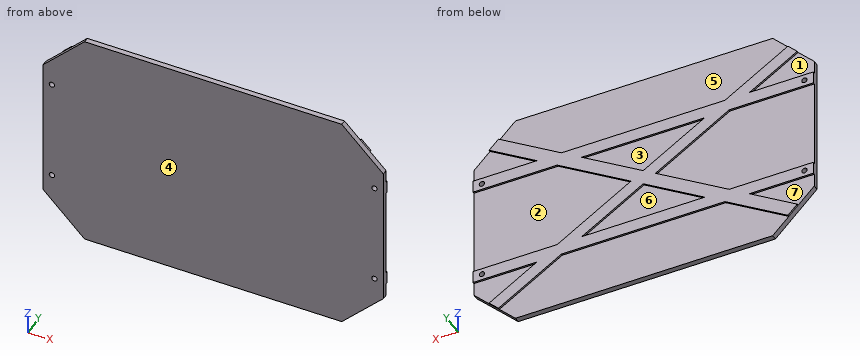
from build123d import *

# Parameters (mm, degrees)
SALIENTE_EXTRUIR1_DEPTH = 3
SALIENTE_EXTRUIR2_DEPTH = 1
CROQUIS3_R              = 1.5
CORTAR_EXTRUIR1_DEPTH   = 115.662203643
CROQUIS5_R              = 1.5
CORTAR_EXTRUIR2_DEPTH   = 115.662203643


with BuildPart() as part:
    # Croquis1 → Saliente-Extruir1 (new body)
    with BuildSketch(Plane(origin=(0, 0, 0), x_dir=(1, 0, 0), z_dir=(0, 1, 0))):
        Polygon((-72.165, -63.334523779), (72.165, -63.334523779), (95.499523779, -40), (95.499523779, 40), (72.165, 63.334523779), (-72.165, 63.334523779), (-95.499523779, 40), (-95.499523779, -40), align=None)
    extrude(amount=SALIENTE_EXTRUIR1_DEPTH)

    # Croquis2 → Saliente-Extruir2 (add)
    with BuildSketch(Plane(origin=(0, 3, 0), x_dir=(1, 0, 0), z_dir=(0, 1, 0))):
        Polygon((-95.499523779, -25.5), (-95.499523779, -32.5), (-59.599057268, -32.5), (-86.448609178, -49.046390822), (-81.218176491, -54.281347289), (-45.874561104, -32.5), (45.875356635, -32.5), (81.215914601, -54.279085399), (86.450579917, -49.048363047), (59.59824255, -32.5), (95.499523779, -32.5), (95.499523779, -25.5), (48.239634992, -25.5), (6.861850317, 0), (48.239634992, 25.5), (95.499523779, 25.5), (95.499523779, 32.5), (59.59824255, 32.5), (86.450579917, 49.048363047), (81.215914601, 54.279085399), (45.875356635, 32.5), (-45.874561104, 32.5), (-81.218176491, 54.281347289), (-86.448609178, 49.046390822), (-59.599057268, 32.5), (-95.499523779, 32.5), (-95.499523779, 25.5), (-48.240274232, 25.5), (-6.861850317, 0), (-48.240274232, -25.5), align=None)
        Polygon((34.516573599, -25.5), (-34.515975042, -25.5), (0, -4.228705845), align=None, mode=Mode.SUBTRACT)
        Polygon((0, 4.228705845), (-34.515975042, 25.5), (34.516573599, 25.5), align=None, mode=Mode.SUBTRACT)
    extrude(amount=SALIENTE_EXTRUIR2_DEPTH)

    # Croquis3 → Cortar-Extruir1 (cut, through all)
    with BuildSketch(Plane(origin=(0, 4, 0), x_dir=(1, 0, 0), z_dir=(0, 1, 0))):
        with Locations(Location((-90.499523779, -29, 0), (0, 0, 270))):
            Circle(CROQUIS3_R)
    extrude(amount=-CORTAR_EXTRUIR1_DEPTH, mode=Mode.SUBTRACT)

    # Croquis5 → Cortar-Extruir2 (cut, through all)
    with BuildSketch(Plane(origin=(0, 4, 0), x_dir=(1, 0, 0), z_dir=(0, 1, 0))):
        with Locations(Location((-90.499523779, 29, 0), (0, 0, 270))):
            Circle(CROQUIS5_R)
        with Locations(Location((90.499523779, 29, 0), (0, 0, 270))):
            Circle(CROQUIS5_R)
        with Locations(Location((90.499523779, -29, 0), (0, 0, 270))):
            Circle(CROQUIS5_R)
    extrude(amount=-CORTAR_EXTRUIR2_DEPTH, mode=Mode.SUBTRACT)


solid = part.part
Source: CAD feature listing. Evaluate the final solid. Frame: model axes, mm. Face numbers are marked on the shaded views. A direction names the side the tool comes from. Round coordinates to 2 decimals unless told otherwise and drop trailing zeros. Order: outer loops, then holes, each group sorted by start corner. A loop starts at its lowest first (then second) coordinate and runs counter-clockwise, first axis right, second up. Notation, with made-up numbers: (-37.75, 5) -> (16.25, 5) arc R23 ccw to (16.25, 31) -> close; hole circle Ø11 at (-35.75, 82). An arc over 180 degrees is marked (long way). Answer as CSV lines item,"result".
Item 1: Reachability of the marked faces 1, 2, 3 and 4 from +Z, -Z, +X, -X, +Y, -Y: full face, straight path, thin tool, end or side. Return the list, or none.
A:
face 1,"-X, +Y"
face 2,"+X, +Y"
face 3,"+Y"
face 4,"+Z, -Z, +X, -X, -Y"
Item 2: Line query: L1, parallel to X at y = 0.8, z = -29; L2, parallel to Z at x = 13.5, y = 3.7; L3, parallel to X at y = 2.7, z = 30. Output: solid intervals per line, ascending.
A:
L1,"-95.5 to -92, -89 to 89, 92 to 95.5"
L2,"-32.5 to -25.5, -12.55 to -4.09, 4.09 to 12.55, 25.5 to 32.5"
L3,"-95.5 to -91.62, -89.38 to 89.38, 91.62 to 95.5"
Item 3: Section A-A, the plane x = -69. Return loops of the section in (y, z).
A:
outline,"(0, -63.33) -> (3, -63.33) -> (3, -46.75) -> (4, -46.75) -> (4, -38.29) -> (3, -38.29) -> (3, -32.5) -> (4, -32.5) -> (4, -25.5) -> (3, -25.5) -> (3, 25.5) -> (4, 25.5) -> (4, 32.5) -> (3, 32.5) -> (3, 38.29) -> (4, 38.29) -> (4, 46.75) -> (3, 46.75) -> (3, 63.33) -> (0, 63.33) -> close"
Item 4: Pull-direction query (X, two-part tool) for the marked faces 5, 6 and 7; classes: pulls with the +X half, pulls with the -X half, needs draft (parallel to the pull), parting line crosses it, or undercut.
A:
face 5,"undercut"
face 6,"undercut"
face 7,"needs draft"
Item 5: Section B-B, the plane y = 1.55. Return loops of the section in (x, z) (3 decimals).
A:
outline,"(-95.5, -40) -> (-72.165, -63.335) -> (72.165, -63.335) -> (95.5, -40) -> (95.5, 40) -> (72.165, 63.335) -> (-72.165, 63.335) -> (-95.5, 40) -> close; hole circle Ø3 at (-90.5, -29); hole circle Ø3 at (-90.5, 29); hole circle Ø3 at (90.5, -29); hole circle Ø3 at (90.5, 29)"
Item 6: Pin query (flat end, axial travel): pin 1 Ø0.8 at (x, y) = (-8.5, 3.5) entering from -Z; pin 2 Ø6.5 at (x, z) = (-82, -41.5) entering from +Y; pin 3 Ø0.8 at (x, y) = (84, 3.5) entering from -Z. Return the tip coordinate at first contact, or that it passes through.
A:
pin 1,"z = -32.5"
pin 2,"y = 3"
pin 3,"z = -51.9"
Item 7: Section C-C, the plane x = 23. Return loops of the section in (y, z), plus the area to 3 significant figures.
A:
outline,"(0, -63.33) -> (3, -63.33) -> (3, -32.5) -> (4, -32.5) -> (4, -25.5) -> (3, -25.5) -> (3, -18.4) -> (4, -18.4) -> (4, -9.95) -> (3, -9.95) -> (3, 9.95) -> (4, 9.95) -> (4, 18.4) -> (3, 18.4) -> (3, 25.5) -> (4, 25.5) -> (4, 32.5) -> (3, 32.5) -> (3, 63.33) -> (0, 63.33) -> close"
area,"411 mm²"
